```python
from build123d import *

# Parameters (mm, degrees)
CHAMFER1_SIZE = 15


with BuildPart() as part:
    # Sweep3: sweep along a path in Sketch1
    with BuildLine(Plane(origin=(0, 0, 0), x_dir=(0, 0, -1), z_dir=(1, 0, 0))) as sweep3_path:
        ThreePointArc((-6.865334795, 25.621778265), (-1.746081847, 13.262808369), (0, 0))
    # Sketch2 → Sweep3 (sweep)
    with BuildSketch(Plane(origin=(0, 0, 0), x_dir=(1, 0, 0), z_dir=(0, 1, 0))):
        with BuildLine():
            Line((3, 22.803508502), (3, 31))
            Line((3, 31), (33, 31))
            Line((33, 31), (33, -31))
            Line((33, -31), (3, -31))
            Line((3, -31), (3, -22.803508502))
            ThreePointArc((3, -22.803508502), (15.901799834, -16.617242913), (22.649503306, -4))
            Line((22.649503306, -4), (25, -4))
            Line((25, -4), (25, 4))
            Line((25, 4), (22.649503306, 4))
            ThreePointArc((22.649503306, 4), (15.901799834, 16.617242913), (3, 22.803508502))
        make_face()
    sweep(path=sweep3_path.line)

    # Chamfer1
    chamfer1_edges = [part.edges().sort_by_distance(p)[0] for p in [
        (33, 5.239417971, 31.689782462),
        (33, 21.286198767, -28.197618768),
    ]]
    chamfer(chamfer1_edges, length=CHAMFER1_SIZE)


solid = part.part
```
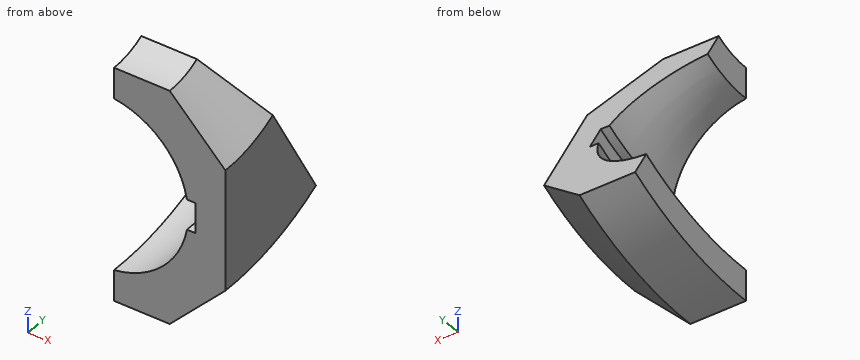
Here's how the part is built. I have some questions about the finished solid (model axes, mm). Give positions to 0.01 mm unless a question says otherwise; leave off trailing zeros. Loops run counter-clockwise (first coordinate to the right, second up) from the corner with the lowest first, then second, coordinate; pieces in that order, holes last. Notation, with made-up numbers: M 25.25,42.25 L 77.25,42.25 A4 cw 77.25,48.25 Z; hole C 68,-39 d8. An arc over 180 degrees is marked long. Use one line per item in the form item = value. Start each with the question number.
Q1. If we section it at C-C (x = 30.5): Write out the boundary of the cut face in (y, z), then the cut area to 3 significant figures.
Q2. If we section it at B-B (x = 20.5): Write out the boundary of the cut face in (y, z).
Q3. If we section it at A-A (x = 5.5): Write out the boundary of the cut face in (y, z), then the cut area to 3 significant figures.
Q4. Will these pins go through, and if not, where does the flat tip stop? pin 1 Ø6 at (x, y) = (13.5, 18) entering from -Z; pin 2 Ø10 at (x, y) = (15.5, 28.5) entering from +Z; pin 3 Ø4 at (x, z) = (6, -12.5) entering from +Y.
Q5. I need wall thicknesses on line 1 along X through (y, z) = (12.5, -2); line 2 along Z through (x, y) = (8, 2.5); line 3 along Z through (x, y) = (17, 11.5). Which ranges of each line are inside material? Lowest first, please.
Taken from the geometry:
q1.outline = M 0,-18.5 A69.74 ccw 34.87,-9.16 L 16.37,22.89 A32.74 cw 0,18.5 Z
q1.area = 993 mm^2
q2.outline = M 0,-28.5 A79.74 ccw 39.87,-17.82 L 30.84,-2.17 A61.67 cw 0,-10.43 Z; M 0,10.43 A40.82 ccw 20.41,15.9 L 11.37,31.55 A22.74 cw 0,28.5 Z
q3.outline = M 0,-31 A82.24 ccw 41.12,-19.98 L 36.79,-12.48 A73.58 cw 0,-22.33 Z; M 0,22.33 A28.91 ccw 14.46,26.21 L 10.12,33.71 A20.24 cw 0,31 Z
q3.area = 465 mm^2
q4.pin_1 = -29.62
q4.pin_2 = -3.13
q4.pin_3 = 37.96
q5.line_1 = 25 to 33
q5.line_2 = -30.96 to -21.52, 21.67 to 31.15
q5.line_3 = -30.19 to -14.49, 17.39 to 31.32
